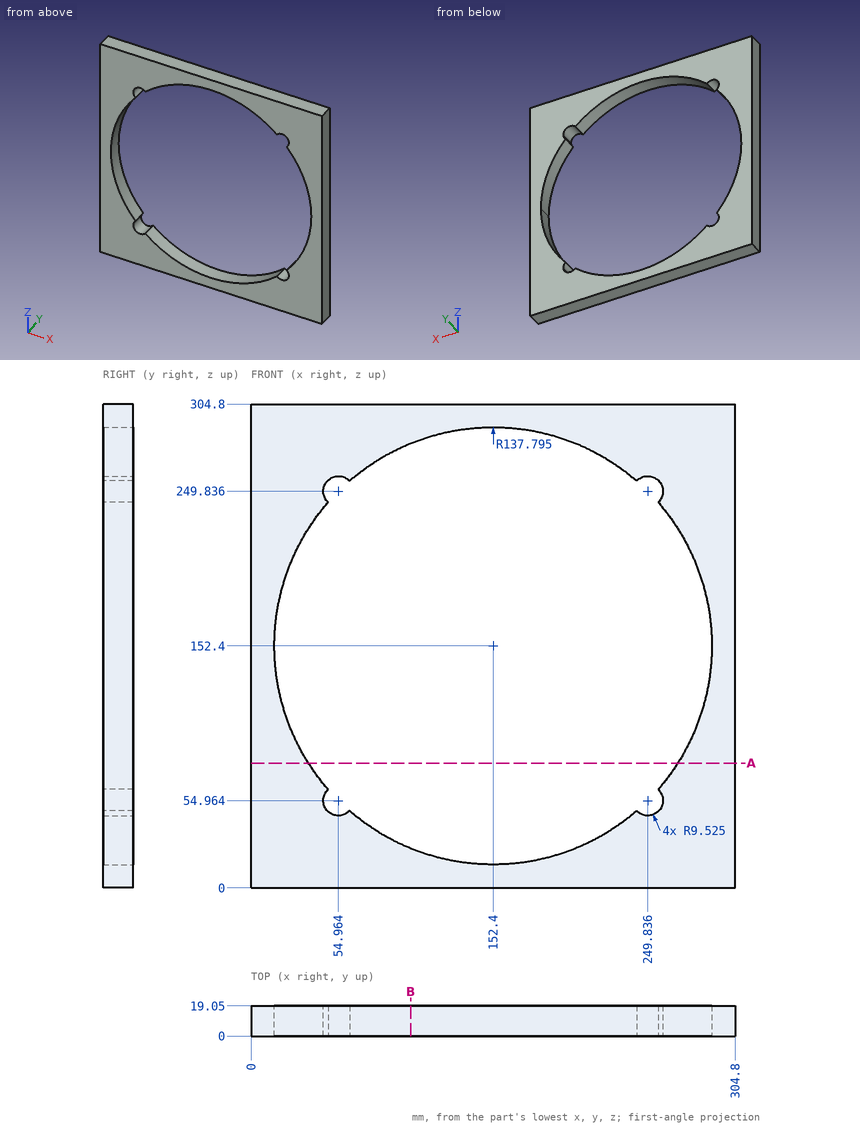
Geometry check sheet. Reference: drawing and pictorial views, mm from the part's lowest x, y, z. Coordinates: 2 decimals unless noted, no trailing zeros. Order: outer loops, then holes, each group sorted by start corner. A loop starts at its lowest first (then second) coordinate and runs counter-clockwise, first axis right, second up. Notation, with made-up numbers: (25, 48.5) -> (60, 48.5) arc R13 ccw to (60, 52.5) -> close; hole circle Ø9 at (47.25, 32). An arc over 180 degrees is marked (long way). Put each result on its own line as item: value. Start each with the question number.
1) Cross-section at A-A (z = 78.5). Enter the section's corners in (x, y).
2) Material ranges on L1, parallel to Z at x = 154, y = 5.5; L2, parallel to Z at x = 155.5, y = 10; L3, parallel to X at y = 14.25, z = 268.5, recorded low to high.
3) Cross-section at B-B (x = 100.5). Enter the section's corners in (y, z).
Geometry check:
1. outline: (0, 0) -> (36.1, 0) -> (36.1, 19.05) -> (0, 19.05) -> close; (268.7, 0) -> (304.8, 0) -> (304.8, 19.05) -> (268.7, 19.05) -> close
2. L1: z = 0 to 14.61, 290.19 to 304.8
2. L2: z = 0 to 14.64, 290.16 to 304.8
2. L3: x = 0 to 78.18, 226.62 to 304.8
3. outline: (0, 0) -> (19.05, 0) -> (19.05, 24.75) -> (0, 24.75) -> close; (0, 280.05) -> (19.05, 280.05) -> (19.05, 304.8) -> (0, 304.8) -> close
